Read the model definition and answer for the solid it produces. Units are mm, in the model's axes. A direction names the side the tool comes from. Coordinates: 2 decimals unless noted, no trailing zeros. Order: outer loops, then holes, each group sorted by start corner. A loop starts at its lowest first (then second) coordinate and runs counter-clockwise, first axis right, second up. Notation, with made-up numbers: (-24.75, 56) - (33.25, 56) arc R22 ccw to (33.25, 83) - close; hole circle Ø11 at (69, 45). An arc over 180 degrees is marked (long way). Use one line per item in the form item = value.
```python
from build123d import *

# Parameters (mm, degrees)
SKETCH4_R            = 55.88
BOSS_EXTRUDE2_DEPTH  = 10.16
BOSS_EXTRUDE4_DEPTH  = 101.6
BOSS_EXTRUDE5_DEPTH  = 9.525
BOSS_EXTRUDE6_START  = -9.525
BOSS_EXTRUDE6_DEPTH  = 9.525
CUT_EXTRUDE4_REACH   = 223.16
SKETCH12_R           = 21.5
SKETCH13_W           = 38.1
SKETCH13_H           = 69.85
CUT_EXTRUDE5_DEPTH   = 76.2
BOSS_EXTRUDE10_DEPTH = 19.05
SKETCH28_R           = 11.2395
CUT_EXTRUDE9_DEPTH   = 38.1
CUT_EXTRUDE10_DEPTH  = 7.366
CHAMFER1_SIZE        = 6.35
SKETCH30_R           = 2.1
CUT_EXTRUDE11_DEPTH  = 7.366
SKETCH31_R           = 3.175
CUT_EXTRUDE12_DEPTH  = 223.900333216
BOSS_EXTRUDE11_DEPTH = 38.1
CHAMFER2_SIZE        = 25.4
CUT_EXTRUDE13_REACH  = 233.204
SKETCH34_R           = 3.175
SKETCH35_R           = 3.175
CUT_EXTRUDE14_DEPTH  = 246.746626534
SKETCH36_W           = 63.5
SKETCH36_H           = 36.709955102
CUT_EXTRUDE15_DEPTH  = 63.5
FILLET1_R            = 6.35
SKETCH37_W           = 210.742334846
SKETCH37_H           = 201.224939079
CUT_EXTRUDE16_DEPTH  = 232.093968202


with BuildPart() as part:
    # Sketch4 → Boss-Extrude2 (new body)
    with BuildSketch(Plane(origin=(0, 0, 0), x_dir=(1, 0, 0), z_dir=(0, 1, 0))):
        with Locations(Location((0, 0, 0), (0, 0, 270))):
            Circle(SKETCH4_R)
    extrude(amount=BOSS_EXTRUDE2_DEPTH)

    # Sketch8 → Boss-Extrude4 (add)
    with BuildSketch(Plane(origin=(0, 10.16, 0), x_dir=(1, 0, 0), z_dir=(0, 1, 0))):
        Polygon((0, 43.994090512), (-38.1, 21.997045256), (-38.1, -21.997045256), (0, -43.994090512), (38.1, -21.997045256), (38.1, 21.997045256), align=None)
    extrude(amount=BOSS_EXTRUDE4_DEPTH)

    # Sketch9 → Boss-Extrude5 (add)
    with BuildSketch(Plane(origin=(-19.05, 0, -32.995567884), x_dir=(-0.8660254037844386, 0, 0.5000000000000003), z_dir=(-0.5000000000000002, 0, -0.8660254037844385))):
        with BuildLine():
            Line((21.997045256, 111.76), (-21.997045256, 111.76))
            Line((-21.997045256, 111.76), (-21.997045256, 124.225996336))
            ThreePointArc((-21.997045256, 124.225996336), (0, 188.144153123), (21.997045256, 124.225996336))
            Line((21.997045256, 124.225996336), (21.997045256, 111.76))
        make_face()
    extrude(amount=-BOSS_EXTRUDE5_DEPTH)

    # Sketch10 → Boss-Extrude6 (add)
    with BuildSketch(Plane(origin=(19.05, 0, 32.995567884), x_dir=(0.8660254037844386, 0, -0.5000000000000001), z_dir=(0.5000000000000001, 0, 0.8660254037844386)).offset(BOSS_EXTRUDE6_START)):
        with BuildLine():
            Line((-21.997045256, 111.76), (21.997045256, 111.76))
            Line((21.997045256, 111.76), (21.997045256, 124.225996336))
            ThreePointArc((21.997045256, 124.225996336), (0, 188.144153123), (-21.997045256, 124.225996336))
            Line((-21.997045256, 124.225996336), (-21.997045256, 111.76))
        make_face()
    extrude(amount=BOSS_EXTRUDE6_DEPTH)

    # Cut-Extrude4: up to this face of the body (flat: up to its plane)
    cut_extrude4_end = Plane(part.part.faces().sort_by_distance((19.05, 104.643172711, 32.995567884))[0])
    # Sketch12 → Cut-Extrude4 (cut, up to the picked face)
    with BuildSketch(Plane(origin=(-19.05, 0, -32.995567884), x_dir=(-0.8660254037844386, 0, 0.5000000000000003), z_dir=(-0.5000000000000002, 0, -0.8660254037844385)), mode=Mode.PRIVATE) as cut_extrude4_sk1:
        with Locations((0, 152.4)):
            Circle(SKETCH12_R)
    cut_extrude4_tool1 = split(extrude(cut_extrude4_sk1.sketch, amount=-CUT_EXTRUDE4_REACH, mode=Mode.PRIVATE), bisect_by=cut_extrude4_end, keep=Keep.BOTH, mode=Mode.PRIVATE)
    add(cut_extrude4_tool1.solids().sort_by(Axis((-19.05, 152.4, -32.995568), (0.5000000000000002, 0, 0.8660254037844385)))[0], mode=Mode.SUBTRACT)

    # Sketch13 → Cut-Extrude5 (cut, symmetric)
    with BuildSketch(Plane(origin=(-19.05, 0, 10.998522628), x_dir=(0.5000000000000002, 0, 0.8660254037844386), z_dir=(-0.8660254037844385, 0, 0.5000000000000001))):
        with Locations((0, 76.835)):
            Rectangle(SKETCH13_W, SKETCH13_H)
    extrude(amount=CUT_EXTRUDE5_DEPTH, both=True, mode=Mode.SUBTRACT)

    # Sketch22 → Boss-Extrude10 (add, symmetric)
    with BuildSketch(Plane(origin=(0, 0, 0), x_dir=(-0.8660254037844386, 0, 0.5000000000000001), z_dir=(-0.5000000000000001, 0, -0.8660254037844386))):
        with BuildLine():
            Line((43.994090512, 41.91), (102.10102108, 41.91))
            ThreePointArc((102.10102108, 41.91), (117.97602108, 26.035), (102.10102108, 10.16))
            Line((102.10102108, 10.16), (43.994090512, 10.16))
            Line((43.994090512, 10.16), (21.997045256, 10.16))
            Line((21.997045256, 10.16), (21.997045256, 41.91))
            Line((21.997045256, 41.91), (43.994090512, 41.91))
        make_face()
    extrude(amount=BOSS_EXTRUDE10_DEPTH, both=True)

    # Sketch28 → Cut-Extrude9 (cut)
    with BuildSketch(Plane(origin=(9.525, 0, 16.497783942), x_dir=(0.8660254037844386, 0, -0.5000000000000001), z_dir=(0.5000000000000001, 0, 0.8660254037844386))):
        with Locations((-102.10102108, 26.035)):
            Circle(SKETCH28_R)
    extrude(amount=-CUT_EXTRUDE9_DEPTH, mode=Mode.SUBTRACT)

    # Sketch29 → Cut-Extrude10 (cut)
    with BuildSketch(Plane(origin=(9.525, 0, 16.497783942), x_dir=(0.8660254037844386, 0, -0.5000000000000001), z_dir=(0.5000000000000001, 0, 0.8660254037844386))):
        with BuildLine():
            Line((-115.737415068, 17.907), (-109.863879848, 17.907))
            ThreePointArc((-109.863879848, 17.907), (-113.34052108, 26.035), (-109.863879848, 34.163))
            Line((-109.863879848, 34.163), (-115.737415068, 34.163))
            ThreePointArc((-115.737415068, 34.163), (-117.97602108, 26.035), (-115.737415068, 17.907))
        make_face()
    extrude(amount=-CUT_EXTRUDE10_DEPTH, mode=Mode.SUBTRACT)

    # Chamfer1
    chamfer1_edges = [part.edges().sort_by_distance(p)[0] for p in [
        (38.1, 41.91, -10.998522628),
        (28.575, 41.91, -27.49630657),
    ]]
    chamfer(chamfer1_edges, length=CHAMFER1_SIZE)

    # Sketch30 → Cut-Extrude11 (cut)
    with BuildSketch(Plane(origin=(0, 41.91, 0), x_dir=(1, 0, 0), z_dir=(0, 1, 0))):
        with Locations(Location((-88.422078008, -51.05051054, 0), (0, 0, 270))):
            Circle(SKETCH30_R)
    extrude(amount=-CUT_EXTRUDE11_DEPTH, mode=Mode.SUBTRACT)

    # Sketch31 → Cut-Extrude12 (cut, through all)
    with BuildSketch(Plane(origin=(0, 10.16, 0), x_dir=(1, 0, 0), z_dir=(0, 1, 0))):
        with Locations(Location((-49.089000823, 6.594762938, 0), (0, 0, 270))):
            Circle(SKETCH31_R)
        with Locations(Location((26.925278647, 41.57222955, 0), (0, 0, 270))):
            Circle(SKETCH31_R)
    cut_extrude12 = extrude(amount=-CUT_EXTRUDE12_DEPTH, mode=Mode.SUBTRACT)

    # Mirror1: Cut-Extrude12 across plane
    add(cut_extrude12.mirror(Plane(origin=(0, 0, 0), x_dir=(-0.8660254037844386, 0, 0.5000000000000001), z_dir=(-0.5000000000000001, 0, -0.8660254037844386))), mode=Mode.SUBTRACT)

    # Sketch33 → Boss-Extrude11 (add)
    with BuildSketch(Plane(origin=(0, 41.91, 0), x_dir=(1, 0, 0), z_dir=(0, 1, 0))):
        with BuildLine():
            Line((-43.411916389, -22.079834386), (-63.092428819, -33.442383535))
            Line((-63.092428819, -33.442383535), (-61.800298466, -35.680418955))
            Line((-61.800298466, -35.680418955), (-60.542722832, -37.858603849))
            Line((-60.542722832, -37.858603849), (-40.91541904, -26.504074545))
            ThreePointArc((-40.91541904, -26.504074545), (-33.742060338, -19.539834386), (-43.411916389, -22.079834386))
        make_face()
    extrude(amount=BOSS_EXTRUDE11_DEPTH)

    # Chamfer2
    chamfer2_edges = [part.edges().sort_by_distance(p)[0] for p in [
        (-61.817575825, 80.01, 35.650493692),
    ]]
    chamfer(chamfer2_edges, length=CHAMFER2_SIZE)

    # Cut-Extrude13: up to this plane
    cut_extrude13_end = Plane(origin=(-60.542722832, 80.01, 37.858603849), z_dir=(-0.500750644235671, 0, -0.8655915851587056))
    # Sketch34 → Cut-Extrude13 (cut, up to the surface)
    with BuildSketch(Plane(origin=(-1.292130352, 0, -2.23803542), x_dir=(-0.8660254037844386, 0, 0.5000000000000003), z_dir=(-0.5000000000000002, 0, -0.8660254037844385)), mode=Mode.PRIVATE) as cut_extrude13_sk1:
        with Locations((55.184849848, 61.159110234)):
            Circle(SKETCH34_R)
    cut_extrude13_tool1 = split(extrude(cut_extrude13_sk1.sketch, amount=-CUT_EXTRUDE13_REACH, mode=Mode.PRIVATE), bisect_by=cut_extrude13_end, keep=Keep.BOTH, mode=Mode.PRIVATE)
    add(cut_extrude13_tool1.solids().sort_by_distance((-49.083612, 61.15911, 25.35439))[0], mode=Mode.SUBTRACT)

    # Sketch35 → Cut-Extrude14 (cut, through all)
    with BuildSketch(Plane(origin=(19.05, 0, 32.995567884), x_dir=(0.8660254037844386, 0, -0.5000000000000001), z_dir=(0.5000000000000001, 0, 0.8660254037844386))):
        with Locations((0, 23.280078313)):
            Circle(SKETCH35_R)
    extrude(amount=-CUT_EXTRUDE14_DEPTH, mode=Mode.SUBTRACT)

    # Sketch36 → Cut-Extrude15 (cut, symmetric)
    with BuildSketch(Plane(origin=(-19.05, 0, 10.998522628), x_dir=(0.5000000000000004, 0, 0.8660254037844384), z_dir=(-0.8660254037844384, 0, 0.5000000000000004))):
        with Locations((0, 174.660846527)):
            Rectangle(SKETCH36_W, SKETCH36_H)
    extrude(amount=CUT_EXTRUDE15_DEPTH, both=True, mode=Mode.SUBTRACT)

    # Fillet1
    # the kernel refuses this fillet: 6.35 mm, written as the material it takes off along each edge
    with BuildSketch(Plane(origin=(12.272597523, 156.305868976, -21.027711652), x_dir=(0.04103819462533737, -0.9988766133891899, -0.023693412713994805), z_dir=(-0.5000000000000003, 0, -0.8660254037844386))) as fillet1_piece_1:
        with BuildLine():
            CenterArc((6.655634068, -6.291985478), FILLET1_R, 97.750867839, 84.965214409)
            Line((0.312767573, -6.592891819), (0, 0))
            ThreePointArc((0, 0), (2.899617679, -0.196427123), (5.799235358, 0))
        make_face()
    extrude(amount=19.675766287, mode=Mode.SUBTRACT)
    with BuildSketch(Plane(origin=(-24.346831236, 156.305868976, 0.114525399), x_dir=(-0.04103819462533767, -0.9988766133891899, 0.023693412713994975), z_dir=(-0.5000000000000003, 0, -0.8660254037844386))) as fillet1_piece_2:
        with BuildLine():
            CenterArc((6.655634068, 6.291985478), FILLET1_R, 177.283917752, 84.965214409)
            Line((0.312767573, 6.592891819), (0, 0))
            ThreePointArc((0, 0), (2.899617679, 0.196427123), (5.799235358, 0))
        make_face()
    extrude(amount=19.675766287, mode=Mode.SUBTRACT)
    with BuildSketch(Plane(origin=(-14.894977291, 156.305868976, 45.261361242), x_dir=(-0.011364190914464473, -0.999913899736612, 0.0065611186835884), z_dir=(-0.5000000000000002, 0, -0.8660254037844386)), Plane(origin=(-36.459231913, 156.305868976, 7.91097661), x_dir=(-0.011364190914463116, -0.999913899736612, 0.0065611186835876165), z_dir=(-0.5000000000000002, 0, -0.8660254037844386))) as fillet1_piece_3:
        with BuildLine():
            CenterArc((6.26760006, -6.320536654), FILLET1_R, 84.478464497, 94.769665105)
            Line((-0.081853204, -6.237210446), (0, 0))
            ThreePointArc((0, 0), (3.439298151, 0.165849191), (6.878596303, 0))
        make_face()
    extrude(amount=20.371490756, mode=Mode.SUBTRACT)
    with BuildSketch(Plane(origin=(25.080722669, 156.305868976, -27.619132734), x_dir=(0.011364190914465366, -0.999913899736612, -0.00656111868358885), z_dir=(-0.5000000000000002, 0, -0.8660254037844386)), Plane(origin=(46.644977291, 156.305868976, 9.731251898), x_dir=(0.011364190914466365, -0.999913899736612, -0.006561118683589426), z_dir=(-0.5000000000000002, 0, -0.8660254037844386))) as fillet1_piece_4:
        with BuildLine():
            CenterArc((6.26760006, 6.320536654), FILLET1_R, 180.751870398, 94.769665105)
            Line((-0.081853204, 6.237210446), (0, 0))
            ThreePointArc((0, 0), (3.439298151, -0.165849191), (6.878596303, 0))
        make_face()
    extrude(amount=20.371490756, mode=Mode.SUBTRACT)

    # Sketch37 → Cut-Extrude16 (cut, through all)
    with BuildSketch(Plane(origin=(0, 0, 0), x_dir=(-0.8660254037844386, 0, 0.5000000000000001), z_dir=(-0.5000000000000001, 0, -0.8660254037844386))):
        with Locations((30.487295463, 97.29801522)):
            Rectangle(SKETCH37_W, SKETCH37_H)
    extrude(amount=CUT_EXTRUDE16_DEPTH, mode=Mode.SUBTRACT)


solid = part.part
```
(1) Given pin 1 Ø5 at (y, z) = (119, 27.5) entering from -X; pin 2 Ø13 at (y, z) = (66.5, 9.5) entering from +X; pin 3 Ø2 at (x, y) = (19, 80) entering from -Z, each flat-ended and moving along its own axis, determine where each tip first touches the part or whether it passes through.
Answer list:
pin_1 = 5.19
pin_2 = 38.1
pin_3 = 10.45
(2) Section B-B, the plane y = 88 is taken. Write down the section's boundary in (x, z), then the cut area to 3 significant figures.
Answer list:
outline = (-19.05, 33) - (38.1, 0) - (38.1, 22) - (0, 43.99) - close
area = 1,050 mm2
(3) Which of the six approach directions +Z, -Z, +X, -X, +Y, -Y give full straight-line access (tool end or side, diameter ignored) to faces 1 (the flat face through (38.1, 49, 5)), 2 (the flat face through (9.12, 73.13, 16.73)), 3 (the flat face through (35.685, 117.906, 17.815)), 4 (the flat face through (-90, 34.163, 70)), 5 (the flat face through (-63, 10.16, 47))?
Answer list:
face_1 = +Z, -Z, +X
face_2 = -Z, +Y
face_3 = -Z, +X
face_4 = +Z, +X
face_5 = +Z, -X, -Y
(4) Section C-C, the plane y = 120 is taken. Write down the section's boundary in (x, z).
Answer list:
outline = (-4.76, 35.75) - (33.34, 13.75) - (38.1, 22) - (0, 43.99) - close
(5) Section A-A, the plane z = -13.5 is taken. Write down the section's boundary in (x, y).
Answer list:
outline = (23.38, 0) - (54.22, 0) - (54.22, 10.16) - (38.1, 10.16) - (38.1, 35.56) - (31.75, 41.91) - (23.38, 41.91) - close
(6) The mould has two halves that part along Y. Classify faces 6 (the flat face through (-47.418, 26.257, 49.374)), 7 (the cylindrical face through (-74.601, 21.73, 54.224)), 8 (the flat face through (-23, 41.91, 24)): +Y half, -Y half, draft (parallel to the pull), parting line (faces both ways), or undercut.
Answer list:
face_6 = draft
face_7 = undercut
face_8 = +Y half
(7) Straight lines are drawn through the part: L1, parallel to Y at x = -1.5, z = 13.5; L2, parallel to X at y = 77.5, z = 32; L3, parallel to X at y = 49, z = 37. For each, find the intervals that lie inside material, in ascending order.
Answer list:
L1 = 0 to 41.91
L2 = -17.33 to 20.77
L3 = -61.04 to -59.06, -12.11 to 12.11
